```python
from build123d import *

# Parameters (mm, degrees)
SKETCH1_R                = 2.5
BOSS_EXTRUDE1_DEPTH      = 5
SKETCH3_W                = 20
SKETCH3_H                = 40
BOSS_EXTRUDE5_DEPTH      = 25
CUT_EXTRUDE2_DEPTH       = 75.20598847
CUT_EXTRUDE2_DEPTH_BACK  = 75.20598847
CUT_EXTRUDE_THIN13_DEPTH = 75.484252037
SKETCH8_W                = 5
SKETCH8_H                = 25
BOSS_EXTRUDE6_DEPTH      = 2
FILLET3_R                = 2
SKETCH9_W                = 5
SKETCH9_H                = 25
BOSS_EXTRUDE7_DEPTH      = 2
FILLET4_R                = 2
SKETCH11_R               = 4.5
CUT_EXTRUDE4_DEPTH       = 25


with BuildPart() as part:
    # Sketch1 → Boss-Extrude1 (new body)
    with BuildSketch(Plane.XY):
        with BuildLine():
            Line((-33.639154819, 54.619565217), (6.360845181, 54.619565217))
            ThreePointArc((6.360845181, 54.619565217), (13.431912992, 51.690633029), (16.360845181, 44.619565217))
            Line((16.360845181, 44.619565217), (16.360845181, -5.380434783))
            ThreePointArc((16.360845181, -5.380434783), (13.431912992, -12.451502594), (6.360845181, -15.380434783))
            Line((6.360845181, -15.380434783), (-33.639154819, -15.380434783))
            ThreePointArc((-33.639154819, -15.380434783), (-40.710222631, -12.451502594), (-43.639154819, -5.380434783))
            Line((-43.639154819, -5.380434783), (-43.639154819, 44.619565217))
            ThreePointArc((-43.639154819, 44.619565217), (-40.710222631, 51.690633029), (-33.639154819, 54.619565217))
        make_face()
        with Locations((3.061250856, 48.159869042)):
            Circle(SKETCH1_R, mode=Mode.SUBTRACT)
        with Locations(Location((3.061250856, -9.840130958, 0), (0, 0, 180))):
            Circle(SKETCH1_R, mode=Mode.SUBTRACT)
        with Locations((-31.938749144, 19.159869042)):
            Circle(SKETCH1_R, mode=Mode.SUBTRACT)
    extrude(amount=BOSS_EXTRUDE1_DEPTH)

    # Sketch3 → Boss-Extrude5 (add)
    with BuildSketch(Plane.XY.offset(5)):
        Polygon((-24.438749144, 44.600432852), (-29.438749144, 44.600432852), (-29.438749144, 37.28199121), (-43.639154819, 37.28199121), (-43.639154819, 32.28199121), (-29.438749144, 32.28199121), (-29.438749144, 7.637328911), (-43.639154819, 7.637328911), (-43.639154819, 2.637328911), (-29.438749144, 2.637328911), (-29.438749144, -5.399567148), (-24.438749144, -5.399567148), (-24.438749144, -15.380434783), (-19.438749144, -15.380434783), (-19.438749144, -5.399567148), (-10.184597354, -5.399567148), (-10.184597354, -15.380434783), (-5.184597354, -15.380434783), (-5.184597354, -5.399567148), (0.561250856, -5.399567148), (0.561250856, 2.637328911), (14.825245568, 2.637328911), (14.825245568, 7.637328911), (0.561250856, 7.637328911), (0.561250856, 17.719700958), (14.825245568, 17.719700958), (14.825245568, 22.719700958), (0.561250856, 22.719700958), (0.561250856, 32.28199121), (14.825245568, 32.28199121), (14.825245568, 37.28199121), (0.561250856, 37.28199121), (0.561250856, 44.600432852), (-5.184597354, 44.600432852), (-5.184597354, 54.581300487), (-10.184597354, 54.581300487), (-10.184597354, 44.600432852), (-19.438749144, 44.600432852), (-19.438749144, 54.581300487), (-24.438749144, 54.581300487), align=None)
        with Locations((-14.438749144, 19.600432852)):
            Rectangle(SKETCH3_W, SKETCH3_H, mode=Mode.SUBTRACT)
    extrude(amount=BOSS_EXTRUDE5_DEPTH)

    # Sketch5 → Cut-Extrude2 (cut, two sides: drawn at the far end of the back side and taken through both)
    with BuildSketch(Plane.XZ.offset(-2.637328911).offset(-CUT_EXTRUDE2_DEPTH_BACK)):
        Polygon((-43.639154819, 30), (-43.639154819, 5), (-29.438749144, 30), align=None)
        Polygon((14.825245568, 30), (0.561250856, 30), (14.825245568, 5), align=None)
    extrude(amount=CUT_EXTRUDE2_DEPTH + CUT_EXTRUDE2_DEPTH_BACK, mode=Mode.SUBTRACT)

    # Sketch7 → Cut-Extrude-Thin13 (cut, through all)
    with BuildSketch(Plane.ZY.offset(24.438749144)):
        Polygon((30, 44.600432852), (5, 54.619565217), (8.72002984, 63.901880553), (33.72002984, 53.882748188), align=None)
        Polygon((5, -15.380434783), (30, -5.399567148), (33.707778838, -14.686782882), (8.707778838, -24.667650517), align=None)
    extrude(amount=-CUT_EXTRUDE_THIN13_DEPTH, mode=Mode.SUBTRACT)

    # Sketch8 → Boss-Extrude6 (add)
    with BuildSketch(Plane.XZ.offset(-39.600432852)):
        with Locations((-15.938749144, 17.5)):
            Rectangle(SKETCH8_W, SKETCH8_H)
    extrude(amount=BOSS_EXTRUDE6_DEPTH)

    # Fillet3
    fillet3_edges = [part.edges().sort_by_distance(p)[0] for p in [
        (-18.438749144, 37.600432852, 17.5),
        (-13.438749144, 37.600432852, 17.5),
    ]]
    fillet(fillet3_edges, radius=FILLET3_R - 0.0001)  # a hair under: the kernel refuses the full size

    # Sketch9 → Boss-Extrude7 (add)
    with BuildSketch(Plane(origin=(0, -0.399567148, 0), x_dir=(1, 0, 0), z_dir=(0, 1, 0))):
        with Locations((-14.690486301, -17.5)):
            Rectangle(SKETCH9_W, SKETCH9_H)
    extrude(amount=BOSS_EXTRUDE7_DEPTH)

    # Fillet4
    fillet4_edges = [part.edges().sort_by_distance(p)[0] for p in [
        (-12.190486301, 1.600432852, 17.5),
        (-17.190486301, 1.600432852, 17.5),
    ]]
    fillet(fillet4_edges, radius=FILLET4_R - 0.0001)  # a hair under: the kernel refuses the full size

    # Sketch11 → Cut-Extrude4 (cut)
    with BuildSketch(Plane.XY.offset(30)):
        with Locations((-31.938749144, 19.159869042)):
            Circle(SKETCH11_R)
    extrude(amount=-CUT_EXTRUDE4_DEPTH, mode=Mode.SUBTRACT)


solid = part.part
```
Part model, mm, in its own coordinate system. A direction names the side the tool comes from. Coordinates: 2 decimals unless noted, no trailing zeros. Write each loop counter-clockwise with the first axis right and the second up, starting at its lowest first coordinate (ties: lowest second). Pieces come first, ordered by that corner, then holes.
Item 1: Slice it at B-B (x = -11). Write the cut outline in (y, z), and give its area (3 significant figures).
Item 2: Slice it at C-C (y = 8.5). Write the cut outline in (x, z), and give its area (3 significant figures).
Item 3: Slice it at D-D (x = 11.5). Write the cut outline in (y, z), and give its area (3 significant figures).
Item 4: Pin check, flat tips, straight feed: pin 1 (6 mm diameter, centred on x = 4.5, y = -6, fed in from +Z); pin 2 (12 mm diameter, centred on x = 9, y = 20, fed in from -Z); pin 3 (0.8 mm diameter, centred on x = -16, z = 16.5, fed in from -Y); pin 4 (8 mm diameter, centred on x = -20.5, z = 20.5, fed in from +Y). Stop position of each tip, or through.
Item 5: Which spindle directions (+Z, -Z, +X, -X, +Y, -Y) get a long thin tool onto all of the face, cutting with end or side? Do faces 1 (the face through (-10.185, 49, 15)), 2 (the face through (-5.185, 48, 15)), 3 (the face through (-15, -5.4, 17)). Say none if no direction does.
Item 6: Probe line 1 (Y direction, x = 1.5, z = 20); line 2 (Y direction, x = -18.5, z = 15); line 3 (X direction, y = -7, z = 25.5). List the from-to ranges inside material, lowest first.
Item 7: Slice it at A-A (y = -8.5). Write the cut outline in (x, z).
Item 8: Mould opens along Y. For faces 4 (the face through (-27, -5.4, 17)), 5 (the face through (-24.439, 49, 15)), 6 (the face through (0.561, 27, 17)), 7 (the face through (6, 32.282, 15)) say: released by +Y, released by -Y, zero draft, split by the parting line, or undercut.
Results found:
1. outline: (-15.38, 0) - (54.62, 0) - (54.62, 5) - (44.6, 5) - (44.6, 30) - (39.6, 30) - (39.6, 5) - (-0.4, 5) - (-0.4, 30) - (-5.4, 30) - (-5.4, 5) - (-15.38, 5) - close
1. area: 600 mm2
2. outline: (-43.64, 0) - (16.36, 0) - (16.36, 5) - (0.56, 5) - (0.56, 30) - (-4.44, 30) - (-4.44, 5) - (-24.44, 5) - (-24.44, 30) - (-29.44, 30) - (-29.44, 5) - (-43.64, 5) - close
2. area: 550 mm2
3. outline: (-13.96, 0) - (53.2, 0) - (53.2, 5) - (37.28, 5) - (37.28, 10.83) - (32.28, 10.83) - (32.28, 5) - (22.72, 5) - (22.72, 10.83) - (17.72, 10.83) - (17.72, 5) - (7.64, 5) - (7.64, 10.83) - (2.64, 10.83) - (2.64, 5) - (-13.96, 5) - close
3. area: 423 mm2
4. pin 1: stops at z = 5
4. pin 2: stops at z = 0
4. pin 3: stops at y = -5.4
4. pin 4: stops at y = 50.01
5. face 1: +Z, +Y
5. face 2: +Z, +X, +Y
5. face 3: +Z, -Y
6. line 1: y = 2.64 to 7.64, 17.72 to 22.72, 32.28 to 37.28
6. line 2: y = -5.4 to -0.4, 39.6 to 44.6
6. line 3: x = -24.44 to -19.44, -10.18 to -5.18
7. outline: (-43.14, 0) - (0.95, 0) - (0.95, 5) - (-5.18, 5) - (-5.18, 22.23) - (-10.18, 22.23) - (-10.18, 5) - (-19.44, 5) - (-19.44, 22.23) - (-24.44, 22.23) - (-24.44, 5) - (-43.14, 5) - close; (5.17, 0) - (15.86, 0) - (15.86, 5) - (5.17, 5) - close
8. face 4: released by -Y
8. face 5: zero draft
8. face 6: undercut
8. face 7: undercut
